The listing builds one solid part. Answer for the finished solid, in the listing's coordinates (mm). A direction names the side the tool comes from. Round coordinates to 2 decimals unless told otherwise and drop trailing zeros. Loops run counter-clockwise (first coordinate to the right, second up) from the corner with the lowest first, then second, coordinate; pieces in that order, holes last. Notation, with made-up numbers: (-10.75, 71) - (14.25, 71) arc R28 ccw to (14.25, 89) - close; hole circle Ø7 at (-1, 22). An arc over 180 degrees is marked (long way). Write item = value, one per line. Start each with the question number.
1) A tool of negligible diameter and unlimited length cuts with its end or side. For faces 1 (the flat face through (-10, 27, -8)), 2 (the cylindrical face through (-1.37, 14.19, -10.41)), 3 (the cylindrical face through (-22.5, 25.5, 0.3)), 4 (the cylindrical face through (16.09, 2.02, 0.72)), from which of +Z, -Z, +X, -X, +Y, -Y can it reach the whole face along a straight path? Write none if from no direction.
2) Given pin 1 Ø0.9 at (y, z) = (26, -24.5) entering from -X; pin 2 Ø9 at (x, z) = (0, 30.078) entering from -Y; pin 3 Ø10 at (x, y) = (-10, 6) entering from -Z; pin 4 Ø1 at (y, z) = (11, 21) entering from +X, each flat-ended and moving along its own axis, determine where each tip first touches the part or whether it passes through.
3) Section A-A, the plane z = 13.8 is taken. Determine the outline of the cut face in (x, y), and give its area (3 significant figures).
4) For a pull along Z with two mould halves and no side action, classify faces 5 (the flat face through (-6, 17, 19)), 6 (the flat face through (8, 4.1, 8)), 7 (the cylindrical face through (-0.607, 25.521, -27.345)) as released by +Z, released by -Z, zero draft, split by the parting line, or undercut.
5) Straight lines are drawn through the part: line 1 along Z through (x, y) = (0, 1); line 2 along Y through (x, z) = (-3, 11.5); line 3 along Z through (x, y) = (0, 26.3). For each, find the intervals that lie inside material, in ascending order.
6) Section B-B, the plane x = -13.8 is taken. Determine the outline of the cut face in (y, z).
7) Section D-D, the plane z = -29 is taken. Determine the outline of the cut face in (x, y), and give its area (3 significant figures).
8) Section C-C, the plane y = 21.5 is taken. Determine the outline of the cut face in (x, z).
Autodesk Inventor part; units mm, degrees
ref_plane "YZ Plane" through (0, 0, 0) normal (1, 0, 0) x (0, 1, 0)
ref_plane "XZ Plane" through (0, 0, 0) normal (0, 1, 0) x (-1, 0, 0)
sketch "Sketch1" plane through (0, 0, 0) normal (0, 0, 1) x (1, 0, 0)
  line L0 (12.525, 32) -> (8, 32)
  line L1 (8, 0) -> (8, 24)
  line L2 (22.5, 27) -> (22.5, 24)
  line L3 (22.5, 24) -> (12.525, 24)
  line L4 (10.5, 0) -> (10.5, 24)
  line L5 (10.5, 32) -> (8, 32)
  line L6 (8, 27) -> (8, 32)
  line L7 (12.525, 27) -> (22.5, 27)
  line L8 (8, 24) -> (8, 27)
  line L9 (12.525, 24) -> (10.5, 24)
  line L10 (12.525, 27) -> (12.525, 32)
  line L11 (8, 0) -> (10.5, 0)
  line L12 (0, -6.4) -> (0, 38.4)
  point P0 (0, 0)
revolve "Revolution1" add sketch "Sketch1" angle 360 about axis through (0, -10, 0) along (0, 1, 0)
sketch "Sketch2" plane through (0, 27, 0) normal (0, 1, 0) x (1, 0, 0)
  line L0 (12.5, 35) -> (-12.5, 35)
  line L1 (-12.5, 35) -> (-12.5, -35)
  line L2 (-12.5, -35) -> (12.5, -35)
  line L3 (12.5, -35) -> (12.5, 35)
  point P0 (0, 0)
  dimension "d8" = 25
  dimension "d9" = 70
extrude "Extrusion1" add sketch "Sketch2" against normal blind 3
sketch "Sketch3" plane through (0, 27, 0) normal (0, 1, 0) x (1, 0, 0)
  circle A0 centre (0, 0) radius 8
extrude "Extrusion2" cut sketch "Sketch3" against normal blind 3
sketch "Sketch4" plane through (-12.5, 27, 35) normal (0, 1, 0) x (1, 0, 0)
  line L0 (12.5, 35) -> (12.5, 65.078)
  line L1 (12.5, 35) -> (12.5, 4.922)
  circle A0 centre (12.5, 65.078) radius 2.8
  circle A1 centre (12.5, 4.922) radius 2.8
  dimension "d14" = 30.078
  dimension "d15" = 30.078
  dimension "d16" = 5.6
  dimension "d17" = 5.6
extrude "Extrusion3" cut sketch "Sketch4" against normal blind 3
sketch "Sketch5" plane through (0, 0, 0) normal (0, -1, 0) x (1, 0, 0)
  line L0 (17.5, 17.5) -> (-17.5, 17.5)
  line L1 (-17.5, 17.5) -> (-17.5, -17.5)
  line L2 (-17.5, -17.5) -> (17.5, -17.5)
  line L3 (17.5, -17.5) -> (17.5, 17.5)
  circle A0 centre (0, 13.8) radius 2.4
  circle A1 centre (13.8, 0) radius 2.4
  circle A2 centre (0, -13.8) radius 2.4
  circle A3 centre (-13.8, 0) radius 2.4
  point P0 (0, 0)
  dimension "d20" = 35
  dimension "d21" = 35
  dimension "d26" = 4.8
  dimension "d28" = 4.8
extrude "Extrusion4" add sketch "Sketch5" against normal blind 4.1
sketch "Sketch6" plane through (17.5, 0, -17.5) normal (0, 0, -1) x (-1, 0, 0)
  point P0 (17.5, 0)
ref_plane "Work Plane1" through (0, 0, 6) normal (0, 0, 1) x (1, 0, 0)
sketch "Sketch7" plane through (0, 0, 6) normal (0, 0, 1) x (1, 0, 0)
  line L0 (-10.5, 24) -> (10.5, 24)
  line L1 (6.5, 24) -> (-6.5, 24)
  line L2 (-6.5, 24) -> (-6.5, 10)
  line L3 (-6.5, 10) -> (6.5, 10)
  line L4 (6.5, 10) -> (6.5, 24)
  point P0 (0, 0)
  dimension "d33" = 13
  dimension "d34" = 14
extrude "Extrusion5" add sketch "Sketch7" along normal blind 13
sketch "Sketch8" plane through (0, 0, 19) normal (0, 0, 1) x (1, 0, 0)
  circle A0 centre (0, 17.1536) radius 5.75
  point P0 (0, 0)
  dimension "d37" = 11.5
extrude "Extrusion6" cut sketch "Sketch8" against normal blind 13
sketch "Sketch9" plane through (0, 4.1, 0) normal (0, 1, 0) x (1, 0, 0)
  circle A0 centre (0, 0) radius 8
extrude "Extrusion7" add sketch "Sketch9" along normal blind 7.2
properties part number "Vacuum Gripper holder"
Geometry check:
q1.face_1 = +Y
q1.face_2 = none
q1.face_3 = -X, +Y
q1.face_4 = -Y
q2.pin_1 = -12.5
q2.pin_2 = 24
q2.pin_3 = -17.5
q2.pin_4 = through
q3.outline = (-17.77, 24) - (-6.5, 24) - (-6.5, 10) - (6.5, 10) - (6.5, 24) - (17.77, 24) - (17.77, 27) - (-17.77, 27) - close; (-17.5, 0) - (-2.4, 0) - (-2.4, 4.1) - (-17.5, 4.1) - close; (2.4, 0) - (17.5, 0) - (17.5, 4.1) - (2.4, 4.1) - close; hole circle Ø11.5 at (0, 17.15)
q3.area = 309 mm2
q4.face_5 = released by +Z
q4.face_6 = zero draft
q4.face_7 = undercut
q5.line_1 = -17.5 to -16.2, -11.4 to 11.4, 16.2 to 17.5
q5.line_2 = 0 to 4.1, 10 to 12.25, 22.06 to 32
q5.line_3 = -35 to -32.88, -27.28 to -8, 8 to 27.28, 32.88 to 35
q6.outline = (0, -17.5) - (4.1, -17.5) - (4.1, -2.4) - (0, -2.4) - close; (0, 2.4) - (4.1, 2.4) - (4.1, 17.5) - (0, 17.5) - close; (24, -17.77) - (27, -17.77) - (27, 17.77) - (24, 17.77) - close
q7.outline = (-12.5, 24) - (-2.58, 24) - (-2.58, 27) - (-12.5, 27) - close; (2.58, 24) - (12.5, 24) - (12.5, 27) - (2.58, 27) - close
q7.area = 59.5 mm2
q8.outline = (-6.5, 8.25) arc R10.5 ccw (long way) to (6.5, 8.25) - (6.5, 19) - (3.76, 19) - (3.76, 6) - (5.29, 6) arc R8 cw (long way) to (-5.29, 6) - (-3.76, 6) - (-3.76, 19) - (-6.5, 19) - close
